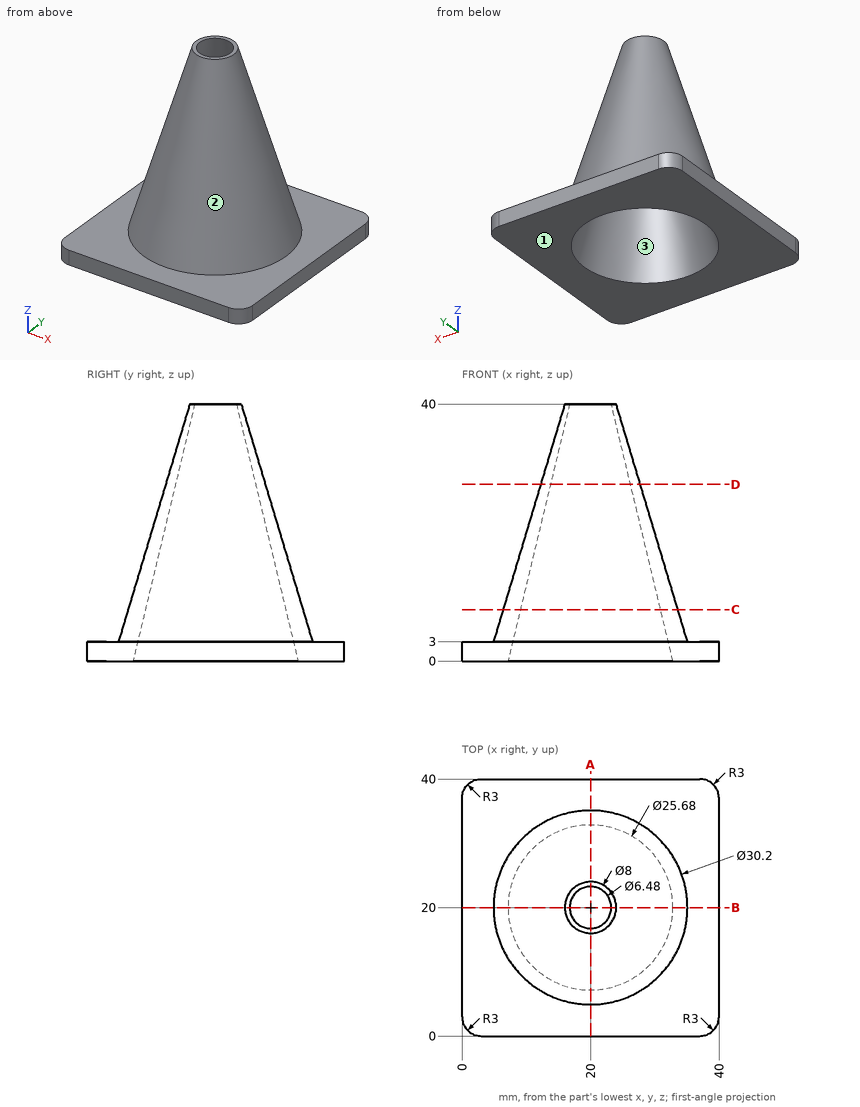
Here's the drawing with two shaded views (mm, measured from the low corner). I have some questions. Coordinates: 2 decimals unless noted, no trailing zeros. Order: outer loops, then holes, each group sorted by start corner. A loop starts at its lowest first (then second) coordinate and runs counter-clockwise, first axis right, second up. Notation, with made-up numbers: M 40.5,31.25 L 99.5,31.25 A16 cw 99.5,37.25 Z; hole C 61,53 d11. An arc over 180 degrees is marked long. Answer as CSV lines item,"result".
Item 1: Imagine slicing it at A-A on x = 20. Write out the boundary of the cut face in (y, z).
Results found:
outline,"M 0,0 L 7.16,0 L 16.76,40 L 16,40 L 4.9,3 L 0,3 Z; M 23.24,40 L 32.84,0 L 40,0 L 40,3 L 35.1,3 L 24,40 Z"
Item 2: Imagine slicing it at D-D on z = 27.5. Write out the boundary of the cut face in (x, y), plus the area to 3 significant figures.
Results found:
outline,"C 20,20 d15.5; hole C 20,20 d12.48"
area,"66.4 mm2"
Item 3: If I drill on line 1 (X direction, y = 15.5, z = 15.5); line 2 (Y direction, x = 18.5, z = 35); line 3 (X direction, y = 20.5, z = 37), over which ranges is the centre line in solid material (lowest first)?
Results found:
line 1,"9.58 to 12.07, 27.93 to 30.42"
line 2,"14.71 to 15.82, 24.18 to 25.29"
line 3,"15.13 to 16.07, 23.93 to 24.87"
Item 4: We'd pull the mould along Y, two halves only. Please class the marked faces 1, 2 and 3: +Y half, -Y half, draft (parallel to the pull), parting line (faces both ways), or undercut.
Results found:
face 1,"draft"
face 2,"parting line"
face 3,"undercut"
Item 5: For pin 1 (1.5 mm diameter, centred on x = 35.5, y = 14, fed in from +Z); pin 2 (1.5 mm diameter, centred on y = 13, z = 27.5, fed in from +X), each with a flat end and sliding along its axis, tell me the tip position at first contact or that it passes through.
Results found:
pin 1,"z = 3"
pin 2,"x = 24.65"
Item 6: Imagine slicing it at C-C on z = 8. Write out the boundary of the cut face in (x, y), plus the area to 3 significant figures.
Results found:
outline,"C 20,20 d27.2; hole C 20,20 d21.84"
area,"206 mm2"
